Check sheet for the modelled part. Datum: model origin and axes. Units: mm. A direction names the side the tool comes from. Round coordinates to 2 decimals unless told otherwise and drop trailing zeros. Write each loop counter-clockwise with the first axis right and the second up, starting at its lowest first coordinate (ties: lowest second). Pieces come first, ordered by that corner, then holes. Notation, with made-up numbers: (25.25, 50.5) - (69.25, 50.5) arc R35 ccw to (69.25, 86.5) - close; hole circle Ø1 at (40.5, 79). An arc over 180 degrees is marked (long way). Use one line per item in the form item = value. Start each with the question number.
1) Section check C-C (y = -36). Record the boundary of the cut face in (x, z).
2) Gauge pin test, flat ends, axial feed: P1, Ø2, axis at y = -17.5, z = -9, coming from the +X side; P2, Ø3, axis at y = 5.5, z = 2.5, coming from the -X side; P3, Ø5, axis at y = 35, z = 19, coming from the +X side; P4, Ø6.5, axis at x = 0, y = 0, coming from the +Z side. Record the tip position at first contact, or that the pin passes through.
3) Section check B-B (z = -11). Record the boundary of the cut face in (x, y), then the cut area to 3 significant figures.
4) Scan lines: probe 1 along Y at (x, z) = (0, -9.5); probe 2 along Z at (x, y) = (-1, -45.5); probe 3 along Y at (x, z) = (-23.5, -18.5). Record each from-to range of solid material in increasing order.
5) Section check A-A (y = 0). Record the boundary of the cut face in (x, z), then the cut area to 3 significant figures.
6) Set-up check for faces 1 (the face through (0, -3, -24)), 2 (the face through (11.923, 3.755, 21.972)), 3 (the face through (11.923, 3.755, -21.972)): record each of +Z, -Z, +X, -X, +Y, -Y from which the full face is reachable in a straight line by a thin tool's end or side.
from build123d import *

# Parameters (mm, degrees)
SKETCH1_R           = 55
BOSS_EXTRUDE1_DEPTH = 20
SKETCH2_R           = 12.5
BOSS_EXTRUDE2_DEPTH = 4
KEYWAY_DEPTH        = 97.269852921


with BuildPart() as part:
    # Sketch1 → Boss-Extrude1 (new, symmetric)
    with BuildSketch(Plane.XY):
        Circle(SKETCH1_R)
    extrude(amount=BOSS_EXTRUDE1_DEPTH, both=True)

    # Sketch2 → Boss-Extrude2 (add)
    with BuildSketch(Plane.XY.offset(20)):
        Circle(SKETCH2_R)
    boss_extrude2 = extrude(amount=BOSS_EXTRUDE2_DEPTH)

    # Mirror1: Boss-Extrude2 across plane
    add(boss_extrude2.mirror(Plane.XY))

    # KeySketch → Keyway (cut, through all)
    with BuildSketch(Plane(origin=(6.62471706, 1.269697251, 24), x_dir=(1, 0, 0), z_dir=(0, 0, 1))):
        with BuildLine():
            ThreePointArc((-7.62471706, 1.021590597), (-6.62471706, -3.769697251), (-5.62471706, 1.021590597))
            ThreePointArc((-5.62471706, 1.021590597), (-6.62471706, 1.230302749), (-7.62471706, 1.021590597))
        make_face()
    extrude(amount=-KEYWAY_DEPTH, mode=Mode.SUBTRACT)


solid = part.part
Results are:
q1.outline = (-41.58, -20) - (41.58, -20) - (41.58, 20) - (-41.58, 20) - close
q2.P1 = 52.47
q2.P2 = -54.85
q2.P3 = 44.37
q2.P4 = 24
q3.outline = circle Ø110 at (0, 0); hole circle Ø5 at (0, 0)
q3.area = 9,480 mm²
q4.probe_1 = -55 to -2.5, 2.5 to 55
q4.probe_2 = -20 to 20
q4.probe_3 = -49.73 to 49.73
q5.outline = (-55, -20) - (-12.5, -20) - (-12.5, -24) - (-2.5, -24) - (-2.5, 24) - (-12.5, 24) - (-12.5, 20) - (-55, 20) - close; (2.5, -24) - (12.5, -24) - (12.5, -20) - (55, -20) - (55, 20) - (12.5, 20) - (12.5, 24) - (2.5, 24) - close
q5.area = 4,360 mm²
q6.face_1 = -Z, +X, -X, +Y, -Y
q6.face_2 = +Z
q6.face_3 = -Z
